from build123d import *

# Parameters (mm, degrees)
F1_DEPTH = 3.175
F2_DEPTH = 9.3218


with BuildPart() as f1:
    # F0 (on Top) → F1 (new body)
    with BuildSketch(Plane.XY):
        with BuildLine():
            ThreePointArc((-9.0909293254, -1.4605), (-9.2065972542, 0.1289311761), (-9.0464659398, 1.7145))
            ThreePointArc((-9.0464659398, 1.7145), (-8.9747244461, 2.0572742564), (-8.89, 2.3970724332))
            Line((-8.89, 2.3970724332), (-8.89, 6.1237182332))
            ThreePointArc((-8.89, 6.1237182332), (-10.2308541629, 3.4440743454), (-10.7834571202, 0.4990766843))
            ThreePointArc((-10.7834571202, 0.4990766843), (-0.2496050755, -10.7921138942), (10.795, 0))
            ThreePointArc((10.795, 0), (10.792113895, 0.2496050431), (10.7834571232, 0.4990766196))
            ThreePointArc((10.7834571232, 0.4990766196), (10.2308541733, 3.4440743147), (8.89, 6.1237182332))
            Line((8.89, 6.1237182332), (8.89, 2.3970724332))
            ThreePointArc((8.89, 2.3970724332), (9.1277798848, 1.2090039806), (9.2075, 0))
            ThreePointArc((9.2075, 0), (0.7325723466, -9.1783110651), (-9.0909293254, -1.4605))
        make_face()
        with BuildLine():
            ThreePointArc((-10.7834571202, 0.4990766843), (-10.2308541629, 3.4440743454), (-8.89, 6.1237182332))
            Line((-8.89, 6.1237182332), (-8.89, 13.97))
            Line((-8.89, 13.97), (-10.16, 13.97))
            Line((-10.16, 13.97), (-10.7834571202, 0.4990766843))
        make_face()
        with BuildLine():
            Line((8.89, 13.97), (8.89, 6.1237182332))
            ThreePointArc((8.89, 6.1237182332), (10.2308541733, 3.4440743147), (10.7834571232, 0.4990766196))
            Line((10.7834571232, 0.4990766196), (10.16, 13.97))
            Line((10.16, 13.97), (8.89, 13.97))
        make_face()
        with BuildLine():
            Line((-8.89, 15.24), (-8.89, 13.97))
            Line((-8.89, 13.97), (0, 13.97))
            Line((0, 13.97), (8.89, 13.97))
            Line((8.89, 13.97), (8.89, 15.24))
            ThreePointArc((8.89, 15.24), (0, 16.0239235845), (-8.89, 15.24))
        make_face()
        Polygon((-10.16, 13.97), (-8.89, 13.97), (-8.89, 15.24), align=None)
        Polygon((8.89, 15.24), (8.89, 13.97), (10.16, 13.97), align=None)
        with BuildLine():
            Line((-8.89, 13.97), (-8.89, 6.1237182332))
            ThreePointArc((-8.89, 6.1237182332), (0, 10.795), (8.89, 6.1237182332))
            Line((8.89, 6.1237182332), (8.89, 13.97))
            Line((8.89, 13.97), (0, 13.97))
            Line((0, 13.97), (-8.89, 13.97))
        make_face()
        with BuildLine():
            Line((-8.89, 6.1237182332), (-8.89, 2.3970724332))
            ThreePointArc((-8.89, 2.3970724332), (0, 9.2075), (8.89, 2.3970724332))
            Line((8.89, 2.3970724332), (8.89, 6.1237182332))
            ThreePointArc((8.89, 6.1237182332), (0, 10.795), (-8.89, 6.1237182332))
        make_face()
        with BuildLine():
            ThreePointArc((8.89, 2.3970724332), (0, 9.2075), (-8.89, 2.3970724332))
            Line((-8.89, 2.3970724332), (-8.89, 1.7145))
            Line((-8.89, 1.7145), (-6.35, 1.7145))
            Line((-6.35, 1.7145), (-6.35, 0))
            Line((-6.35, 0), (-3.4925, 0))
            ThreePointArc((-3.4925, 0), (0, 3.4925), (3.4925, 0))
            Line((3.4925, 0), (8.89, 0))
            Line((8.89, 0), (8.89, 2.3970724332))
        make_face()
        with BuildLine():
            Line((-6.35, -1.4605), (-9.0909293254, -1.4605))
            ThreePointArc((-9.0909293254, -1.4605), (0.7325723466, -9.1783110651), (9.2075, 0))
            ThreePointArc((9.2075, 0), (9.1277798848, 1.2090039806), (8.89, 2.3970724332))
            Line((8.89, 2.3970724332), (8.89, 0))
            Line((8.89, 0), (3.4925, 0))
            ThreePointArc((3.4925, 0), (0, -3.4925), (-3.4925, 0))
            Line((-3.4925, 0), (-6.35, 0))
            Line((-6.35, 0), (-6.35, -1.4605))
        make_face()
        with BuildLine():
            ThreePointArc((-8.89, 2.3970724332), (-8.9747244461, 2.0572742564), (-9.0464659398, 1.7145))
            Line((-9.0464659398, 1.7145), (-8.89, 1.7145))
            Line((-8.89, 1.7145), (-8.89, 2.3970724332))
        make_face()
    extrude(amount=-F1_DEPTH)

    # F0 (on Top) → F2 (join)
    with BuildSketch(Plane.XY):
        with BuildLine():
            ThreePointArc((-10.7834571202, 0.4990766843), (-10.2308541629, 3.4440743454), (-8.89, 6.1237182332))
            Line((-8.89, 6.1237182332), (-8.89, 13.97))
            Line((-8.89, 13.97), (-10.16, 13.97))
            Line((-10.16, 13.97), (-10.7834571202, 0.4990766843))
        make_face()
        with BuildLine():
            ThreePointArc((-9.0909293254, -1.4605), (-9.2065972542, 0.1289311761), (-9.0464659398, 1.7145))
            ThreePointArc((-9.0464659398, 1.7145), (-8.9747244461, 2.0572742564), (-8.89, 2.3970724332))
            Line((-8.89, 2.3970724332), (-8.89, 6.1237182332))
            ThreePointArc((-8.89, 6.1237182332), (-10.2308541629, 3.4440743454), (-10.7834571202, 0.4990766843))
            ThreePointArc((-10.7834571202, 0.4990766843), (-0.2496050755, -10.7921138942), (10.795, 0))
            ThreePointArc((10.795, 0), (10.792113895, 0.2496050431), (10.7834571232, 0.4990766196))
            ThreePointArc((10.7834571232, 0.4990766196), (10.2308541733, 3.4440743147), (8.89, 6.1237182332))
            Line((8.89, 6.1237182332), (8.89, 2.3970724332))
            ThreePointArc((8.89, 2.3970724332), (9.1277798848, 1.2090039806), (9.2075, 0))
            ThreePointArc((9.2075, 0), (0.7325723466, -9.1783110651), (-9.0909293254, -1.4605))
        make_face()
        with BuildLine():
            Line((8.89, 13.97), (8.89, 6.1237182332))
            ThreePointArc((8.89, 6.1237182332), (10.2308541733, 3.4440743147), (10.7834571232, 0.4990766196))
            Line((10.7834571232, 0.4990766196), (10.16, 13.97))
            Line((10.16, 13.97), (8.89, 13.97))
        make_face()
        with BuildLine():
            Line((-8.89, 15.24), (-8.89, 13.97))
            Line((-8.89, 13.97), (0, 13.97))
            Line((0, 13.97), (8.89, 13.97))
            Line((8.89, 13.97), (8.89, 15.24))
            ThreePointArc((8.89, 15.24), (0, 16.0239235845), (-8.89, 15.24))
        make_face()
        Polygon((-10.16, 13.97), (-8.89, 13.97), (-8.89, 15.24), align=None)
        Polygon((8.89, 15.24), (8.89, 13.97), (10.16, 13.97), align=None)
    extrude(amount=F2_DEPTH)


solid = f1.part
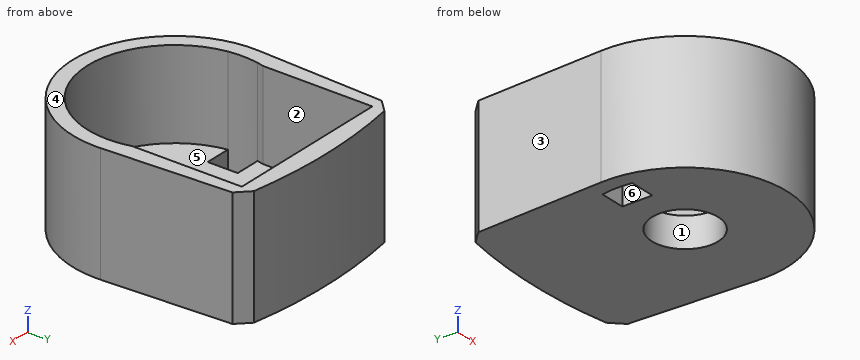
For this review, take the finished solid that the model builds, in its own axes (mm). Face numbers are marked on the shaded views. A direction names the side the tool comes from. Give positions to 0.01 mm unless a question says otherwise; leave off trailing zeros. Loops run counter-clockwise (first coordinate to the right, second up) from the corner with the lowest first, then second, coordinate; pieces in that order, holes last.
Item 1: Tool access review of the marked faces 1 and 2: name each direction out of +Z, -Z, +X, -X, +Y, -Y from which nothing blocks a thin tool from reaching the whole face with its end or side.
Item 2: Take a section at D-D, the plane y = -5.75. State the section outline as (x, z) points (3 decimals).
Item 3: Take a section at B-B, the plane z = 2.5. State the section outline as (x, y) points (1 decimal), and give its area (3 significant figures).
Item 4: For line 1 along Y through (x, z) = (0, -1.65) (1 decimal); line 2 along X through (y, z) = (-1, -2.5); line 3 along Z through (x, y) = (-4.25, -2.75) (3 decimals), list the stretches that pass through material, from the lowest coordinate up.
Item 5: Take a section at A-A, the plane x = 0. State the section outline as (y, z) points (1 decimal).
Item 6: Take a section at C-C, the plane x = -7. State the section outline as (y, z) points (1 decimal).
Item 7: Insertion check: pin 1 (1.4 mm diameter, centred on x = -8, z = -1.5, fed in from +Y); pin 2 (3 mm diameter, centred on y = 8, z = 5.5, fed in from -X); pin 3 (3 mm diameter, centred on x = 4, z = 4.5, fed in from -Y). Each pin has a flat end and moves straight along its axis. Give the tip position at first contact, or say it passes through.
Item 8: Draft analysis for pull direction Y (two halves, no side actions). For the marked faces 3, 4, 5 and 6, state which applies: +Y half, -Y half, draft (parallel to the pull), parting line (faces both ways), or undercut.
Calculated:
1. face 1: +Z, -Z
1. face 2: +Z
2. outline: (-9.136, -3.175) - (9.136, -3.175) - (9.136, 9.322) - (7.191, 9.322) - (7.191, 0) - (-7.191, 0) - (-7.191, 9.322) - (-9.136, 9.322) - close
3. outline: (-10.8, 0.5) arc R10.8 ccw (long way) to (10.8, 0.5) - (10.2, 14) - (8.9, 15.2) arc R50.8 ccw to (-8.9, 15.2) - (-10.2, 14) - close; hole (-8.9, 2.4) arc R9.2 ccw (long way) to (8.9, 2.4) - (8.9, 14) - (-8.9, 14) - close
3. area: 127 mm2
4. line 1: y = -10.8 to -3.5, 3.5 to 16
4. line 2: x = -10.75 to -9.15, -6.35 to -3.35, 3.35 to 10.75
4. line 3: z = -3.175 to 0
5. outline: (-10.8, -3.2) - (-3.5, -3.2) - (-3.5, 0) - (-9.2, 0) - (-9.2, 9.3) - (-10.8, 9.3) - close; (3.5, -3.2) - (16, -3.2) - (16, 9.3) - (14, 9.3) - (14, 0) - (3.5, 0) - close
6. outline: (-8.2, -3.2) - (-1.5, -3.2) - (-1.5, 0) - (-6, 0) - (-6, 9.3) - (-8.2, 9.3) - close; (1.7, -3.2) - (15.5, -3.2) - (15.5, 9.3) - (14, 9.3) - (14, 0) - (1.7, 0) - close
7. pin 1: stops at y = 15.5
7. pin 2: stops at x = -10.51
7. pin 3: stops at y = -10.5
8. face 3: +Y half
8. face 4: draft
8. face 5: undercut
8. face 6: undercut
